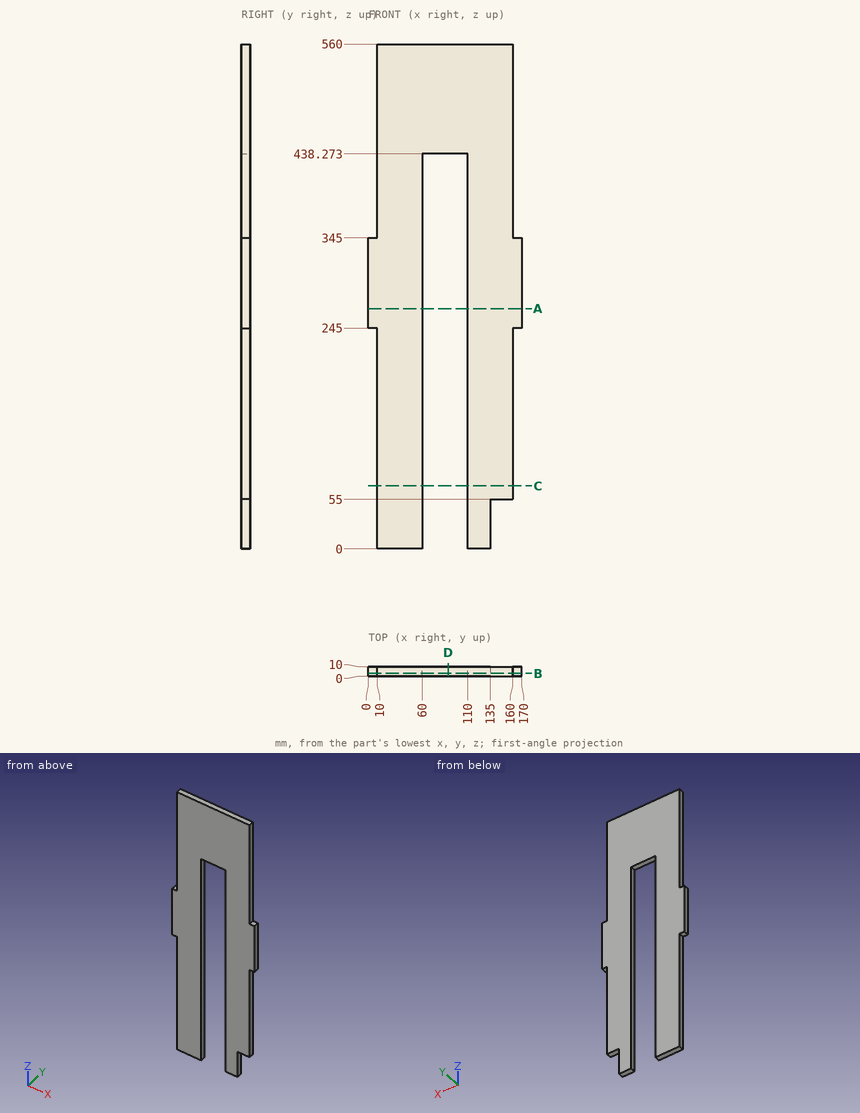
Source: three-view drawing plus pictorial views. Frame: mm from the lowest corner of the part. Round coordinates to 2 decimals unless told otherwise and drop trailing zeros. Order: outer loops, then holes, each group sorted by start corner. A loop starts at its lowest first (then second) coordinate and runs counter-clockwise, first axis right, second up. Notation, with made-up numbers: (-35.75, 19) -> (-2.75, 19) arc R8 cw to (-2.75, 30) -> close; hole circle Ø6 at (32.5, 42). An arc over 180 degrees is marked (long way). Use one line per item in the form item = value. Start each with the question number.
1. Line query: probe 1 along X at (y, z) = (2.75, 354.5); probe 2 along X at (y, z) = (2.5, 342.5); probe 3 along Z at (x, y) = (84.5, 5). Output: solid intervals per line, ascending.
2. Cut plane D-D (x = 88.5). Return the cut outline in (y, z), then the cut area to 3 significant figures.
3. Cut plane B-B (y = 3). Return the cut outline in (x, z), then the cut area to 3 significant figures.
4. Pin query (flat end, axial travel): pin 1 Ø3 at (x, y) = (167, 6.5) entering from -Z; pin 2 Ø3 at (y, z) = (2.5, 404.5) entering from +X; pin 3 Ø3 at (y, z) = (3, 498) entering from -X. Return the tip coordinate at first contact, or that it passes through.
5. Cut plane A-A (z = 266.5). Return the cut outline in (x, y), then the cut area to 3 significant figures.
6. Cut plane C-C (z = 70). Return the cut outline in (x, y).
Solution:
q1.probe_1 = 10 to 60, 110 to 160
q1.probe_2 = 0 to 60, 110 to 170
q1.probe_3 = 438.27 to 560
q2.outline = (0, 438.27) -> (10, 438.27) -> (10, 560) -> (0, 560) -> close
q2.area = 1,220 mm^2
q3.outline = (0, 245) -> (10, 245) -> (10, 0) -> (60, 0) -> (60, 438.27) -> (110, 438.27) -> (110, 0) -> (135, 0) -> (135, 55) -> (160, 55) -> (160, 245) -> (170, 245) -> (170, 345) -> (160, 345) -> (160, 560) -> (10, 560) -> (10, 345) -> (0, 345) -> close
q3.area = 62,700 mm^2
q4.pin_1 = 245
q4.pin_2 = 160
q4.pin_3 = 10
q5.outline = (0, 0) -> (60, 0) -> (60, 10) -> (0, 10) -> close; (110, 0) -> (170, 0) -> (170, 10) -> (110, 10) -> close
q5.area = 1,200 mm^2
q6.outline = (10, 0) -> (60, 0) -> (60, 10) -> (10, 10) -> close; (110, 0) -> (160, 0) -> (160, 10) -> (110, 10) -> close
